Source: three-view drawing plus pictorial views. Frame: mm from the lowest corner of the part. A direction names the side the tool comes from. Coordinates: 2 decimals unless noted, no trailing zeros. Write each loop counter-clockwise with the first axis right and the second up, starting at its lowest first coordinate (ties: lowest second). Pieces come first, ordered by that corner, then holes. Notation, with made-up numbers: (-39.5, 26.25) - (-4.5, 26.25) arc R26 cw to (-4.5, 56.25) - close; hole circle Ø11 at (-29.75, 9.25). An arc over 180 degrees is marked (long way). One line per item, written item: value.
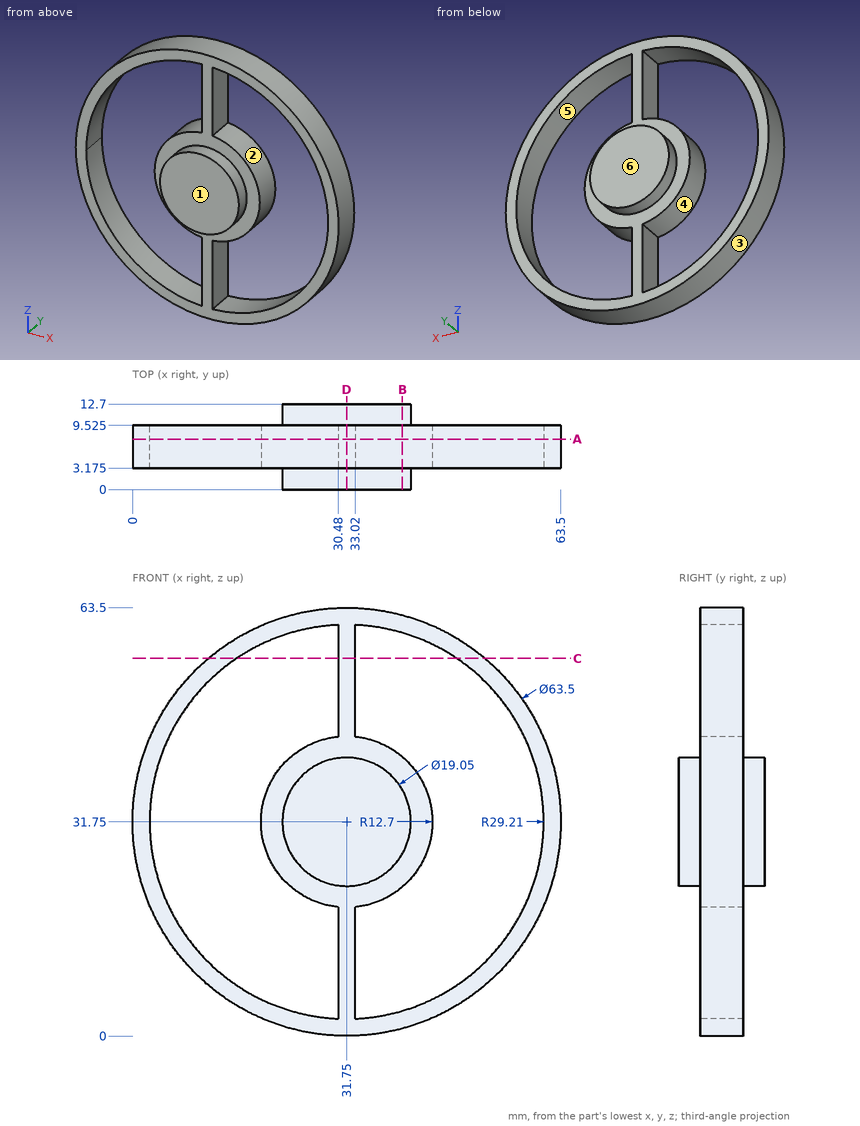
1) Section query C-C on z = 56. Output: boundary loops of the cut face in (x, y) (3 decimals), then the cut area to 3 significant figures.
Values found:
outline: (11.256, 3.175) - (15.466, 3.175) - (15.466, 9.525) - (11.256, 9.525) - close; (30.48, 3.175) - (33.02, 3.175) - (33.02, 9.525) - (30.48, 9.525) - close; (48.034, 3.175) - (52.244, 3.175) - (52.244, 9.525) - (48.034, 9.525) - close
area: 69.6 mm2
2) Section query A-A on y = 7.5. Output: boundary loops of the cut face in (x, z).
Values found:
outline: circle Ø63.5 at (31.75, 31.75); hole (30.48, 2.57) - (30.48, 19.11) arc R12.7 cw to (30.48, 44.39) - (30.48, 60.93) arc R29.21 ccw to start; hole (33.02, 2.57) arc R29.21 ccw to (33.02, 60.93) - (33.02, 44.39) arc R12.7 cw to (33.02, 19.11) - close
3) Material intervals for line 1 (X direction, y = 8, z = 14); line 2 (X direction, y = 6.5, z = 46.5); line 3 (Y direction, x = 58, z = 17.5) (3 decimals), sorted ascending.
Values found:
line 1: 5.43 to 8.55, 30.48 to 33.02, 54.95 to 58.07
line 2: 3.63 to 6.54, 30.48 to 33.02, 56.96 to 59.87
line 3: 3.175 to 9.525
4) Section query B-B on x = 40. Output: boundary loops of the cut face in (y, z) (3 decimals).
Values found:
outline: (0, 26.989) - (3.175, 26.989) - (3.175, 22.095) - (9.525, 22.095) - (9.525, 26.989) - (12.7, 26.989) - (12.7, 36.511) - (9.525, 36.511) - (9.525, 41.405) - (3.175, 41.405) - (3.175, 36.511) - (0, 36.511) - close; (3.175, 1.091) - (9.525, 1.091) - (9.525, 3.729) - (3.175, 3.729) - close; (3.175, 59.771) - (9.525, 59.771) - (9.525, 62.409) - (3.175, 62.409) - close
5) Draft query along Z for the marked faces 3, 4, 5 and 6. Return one class per face: released by +Z, released by -Z, zero draft, split by the parting line, or undercut.
Values found:
face 3: split by the parting line
face 4: undercut
face 5: undercut
face 6: zero draft
6) Section query D-D on x = 31.75. Output: boundary loops of the cut face in (y, z) (3 decimals).
Values found:
outline: (0, 22.225) - (3.175, 22.225) - (3.175, 0) - (9.525, 0) - (9.525, 22.225) - (12.7, 22.225) - (12.7, 41.275) - (9.525, 41.275) - (9.525, 63.5) - (3.175, 63.5) - (3.175, 41.275) - (0, 41.275) - close
7) Contact query for flat-ended pins moving along their axis: P1, Ø12, axis at x = 17.5, z = 52.5, coming from the +Y side (3 decimals); P2, Ø7, axis at y = 7.5, z = 55, coming from the +X side; P3, Ø1.5, axis at x = 35.5, y = 2.5, coming from the +Z side. Output: stop coordinate, or through.
Values found:
P1: y = 9.525
P2: x = 56.61
P3: z = 63.31
8) Reachability of the marked faces 1 and 2 from +Z, -Z, +X, -X, +Y, -Y: full face, straight path, thin tool, end or side. Return the list, or none.
Values found:
face 1: +Z, -Z, +X, -X, -Y
face 2: +Y, -Y
